```python
from build123d import *

# Parameters (mm, degrees)
F1_DEPTH = 25.4
F2_DEPTH = 25.4
F3_R     = 9.9934379812
F4_DEPTH = 25.4


with BuildPart() as f1:
    # F0 (on Front) → F1 (new body)
    with BuildSketch(Plane.XZ):
        with BuildLine():
            Line((-122.5946694613, 43.2584390598), (-122.5946694613, 56.6831417382))
            Line((-122.5946694613, 56.6831417382), (-109.1699667829, 56.6831417382))
            ThreePointArc((-109.1699667829, 56.6831417382), (-132.0873677605, 66.1758400375), (-122.5946694613, 43.2584390598))
        make_face()
        with BuildLine():
            Line((-109.1699667829, 56.6831417382), (-122.5946694613, 56.6831417382))
            Line((-122.5946694613, 56.6831417382), (-122.5946694613, 43.2584390598))
            ThreePointArc((-122.5946694613, 43.2584390598), (-113.101971162, 47.1904434389), (-109.1699667829, 56.6831417382))
        make_face()
        with BuildLine():
            Line((-45.4307209175, 56.6831417382), (-109.1699667829, 56.6831417382))
            ThreePointArc((-109.1699667829, 56.6831417382), (-113.101971162, 47.1904434389), (-122.5946694613, 43.2584390598))
            Line((-122.5946694613, 43.2584390598), (-122.5946694613, 5.5007226765))
            Line((-122.5946694613, 5.5007226765), (-32.0475660264, 5.5007226765))
            Line((-32.0475660264, 5.5007226765), (-32.0475660264, 43.2999868471))
            ThreePointArc((-32.0475660264, 43.2999868471), (-41.5108856036, 47.2198221611), (-45.4307209175, 56.6831417382))
        make_face()
        with BuildLine():
            ThreePointArc((-18.6644111354, 56.6831417382), (-32.0475660264, 70.0662966292), (-45.4307209175, 56.6831417382))
            Line((-45.4307209175, 56.6831417382), (-32.0475660264, 56.6831417382))
            Line((-32.0475660264, 56.6831417382), (-32.0475660264, 43.2999868471))
            ThreePointArc((-32.0475660264, 43.2999868471), (-22.5842464493, 47.2198221611), (-18.6644111354, 56.6831417382))
        make_face()
        with BuildLine():
            Line((-32.0475660264, 56.6831417382), (-45.4307209175, 56.6831417382))
            ThreePointArc((-45.4307209175, 56.6831417382), (-41.5108856036, 47.2198221611), (-32.0475660264, 43.2999868471))
            Line((-32.0475660264, 43.2999868471), (-32.0475660264, 56.6831417382))
        make_face()
    extrude(amount=F1_DEPTH)

    # F2 (add): a face of the model
    f2_faces = [f1.faces().sort_by_distance(p)[0] for p in [
        (-77.3003438502, -12.7, 56.6831417382),
    ]]
    extrude(f2_faces, amount=F2_DEPTH)

    # F3 (on face) → F4 (join)
    with BuildSketch(Plane.XZ.offset(25.4)):
        with Locations((-32.0475660264, 56.6831417382)):
            Circle(F3_R)
    extrude(amount=-F4_DEPTH)


solid = f1.part
```
Verification items for the finished model (mm, model axes). A direction names the side the tool comes from. Coordinates: 2 decimals unless noted, no trailing zeros. Loops run counter-clockwise (first coordinate to the right, second up) from the corner with the lowest first, then second, coordinate; pieces in that order, holes last. Notation, with made-up numbers: (77.5, 39) -> (135.5, 39) arc R18 ccw to (135.5, 57) -> close; hole circle Ø7 at (21, -0.5). An arc over 180 degrees is marked (long way). Answer in a Markdown table with one row per item.
1) Section check C-C (z = 30). Record the cut outline in (x, y).
The answers:
| item | result |
|---|---|
| outline | (-122.59, -25.4) -> (-32.05, -25.4) -> (-32.05, 0) -> (-122.59, 0) -> close |
2) Draft check along X on faces 3 (the face through (-122.595, -13, 25)), 4 (the face through (-131.769, -12.522, 66.484)), 5 (the face through (-77, -13, 82.083)). Enter one of: released by +X, released by -X, zero draft, split by the parting line, or undercut.
The answers:
| item | result |
|---|---|
| face 3 | released by -X |
| face 4 | undercut |
| face 5 | zero draft |
3) Section check B-B (z = 61). Record the cut outline in (x, y).
The answers:
| item | result |
|---|---|
| outline | (-135.31, -25.4) -> (-109.88, -25.4) -> (-109.88, 0) -> (-135.31, 0) -> close; (-109.17, -25.4) -> (-45.43, -25.4) -> (-45.43, 0) -> (-109.17, 0) -> close; (-44.72, -25.4) -> (-19.38, -25.4) -> (-19.38, 0) -> (-44.72, 0) -> close |
4) Section check A-A (y = -20). Record the cut outline in (x, z), and give its area (3 significant figures).
The answers:
| item | result |
|---|---|
| outline | (-122.59, 5.5) -> (-32.05, 5.5) -> (-32.05, 43.3) arc R13.38 ccw (long way) to (-45.43, 56.68) -> (-45.43, 82.08) -> (-109.17, 82.08) -> (-109.17, 56.68) arc R13.42 ccw (long way) to (-122.59, 43.26) -> close |
| area | 7,100 mm2 |
5) Access from +Z, -Z, +X, -X, +Y, -Y to the whole of each face (thin tool, end or side, straight path). Record for faces 1 (the face through (-32.048, -13, 24)), 2 (the face through (-77, -25.4, 43)).
The answers:
| item | result |
|---|---|
| face 1 | -Z, +X, +Y, -Y |
| face 2 | +Z, -Z, +X, -X, -Y |
6) Section check D-D (x = -41). Record the cut outline in (y, z), and give its area (3 significant figures).
The answers:
| item | result |
|---|---|
| outline | (-25.4, 5.5) -> (0, 5.5) -> (0, 66.63) -> (-25.4, 66.63) -> close |
| area | 1,550 mm2 |
7) Depth check by flat-ended pin: P1, Ø6, axis at x = -106, z = 58, coming from the +Y side; P2, Ø5, axis at y = -17, z = 30.5, coming from the +X side; P3, Ø3, axis at x = -34.5, y = -14, coming from the +Z side; P4, Ø7.5, axis at y = -7.5, z = 70.5, coming from the -X side. Enter the tip coordinate at first touch or a pass-through.
The answers:
| item | result |
|---|---|
| P1 | stops at y = 0 |
| P2 | stops at x = -32.05 |
| P3 | stops at z = 70.03 |
| P4 | stops at x = -131.48 |
8) Scan lines: line 1 along X through (y, z) = (-11, 60); line 2 along X through (y, z) = (-21, 63.5); line 3 along X through (y, z) = (-19, 21). Record each from-to range of solid material in increasing order. Write a range as from..to.
The answers:
| item | result |
|---|---|
| line 1 | x = -135.6..-109.59, -109.17..-45.43, -45.01..-19.08 |
| line 2 | x = -134.16..-111.03, -109.17..-45.43, -43.56..-20.53 |
| line 3 | x = -122.59..-32.05 |
